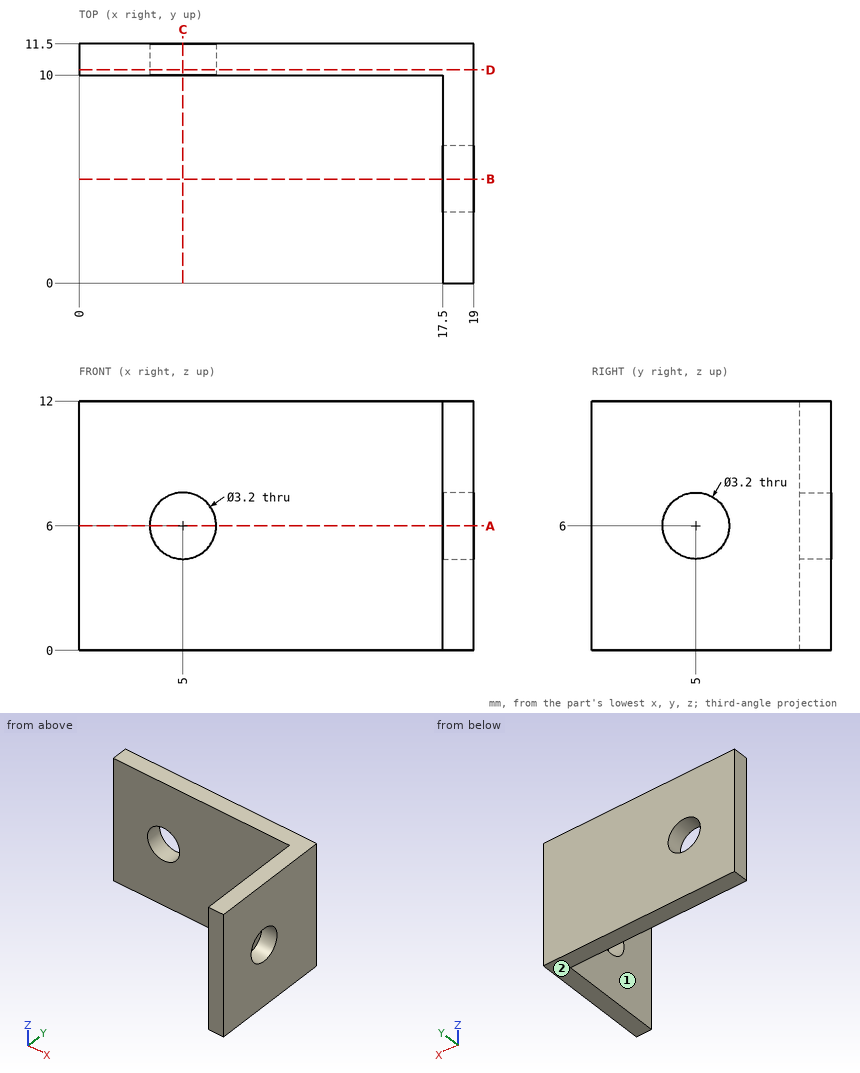
Part print with two shaded views. Sizes in mm from the minimum x, y, z corner. A direction names the side the tool comes from. Round coordinates to 2 decimals unless told otherwise and drop trailing zeros. Order: outer loops, then holes, each group sorted by start corner. A loop starts at its lowest first (then second) coordinate and runs counter-clockwise, first axis right, second up. Notation, with made-up numbers: M 83,11.25 L 128,11.25 A27 cw 128,35.25 Z; hole C -26,79 d4. An arc over 180 degrees is marked long. Answer in a Markdown table with one row per item. Add a question column.
Q1. 3-axis set-ups, long thin cutter, end or side, ignore diameter. For the marked faces 1 and 2: which of +Z, -Z, +X, -X, +Y, -Y reach the whole face in a straight line?
Q2. Wall check: L1, parallel to Z at x = 5, y = 10.6; L2, parallel to Y at x = 18.55, z = 6; L3, parallel to Y at x = 9, z = 5.5. Give the ranges that are in metal, low to high. Write a range as from..to.
Q3. Cut at A-A on z = 6. Give the cut face in (x, y).
Q4. Cut at C-C on x = 5. Give the cut face in (y, z), and give its area (3 significant figures).
Q5. Pin check, flat tips, straight feed: pin 1 (4 mm diameter, centred on x = 2, z = 4.5, fed in from -Y); pin 2 (3 mm diameter, centred on y = 3, z = 5, fed in from -X). Stop position of each tip, or through.
Q6. Cut at B-B on y = 5. Give the cut face in (x, z), and give its area (3 significant figures).
Q7. Cut at D-D on y = 10.25. Give the cut face in (x, z), and give its area (3 significant figures).
Established:
| question | item | result |
|---|---|---|
| 1 | face 1 | +Z, -Z, -X, -Y |
| 1 | face 2 | -Z, +X, -X, +Y, -Y |
| 2 | L1 | z = 0..4.4, 7.6..12 |
| 2 | L2 | y = 0..3.4, 6.6..11.5 |
| 2 | L3 | y = 10..11.5 |
| 3 | outline | M 0,10 L 3.4,10 L 3.4,11.5 L 0,11.5 Z; M 6.6,10 L 17.5,10 L 17.5,6.6 L 19,6.6 L 19,11.5 L 6.6,11.5 Z; M 17.5,0 L 19,0 L 19,3.4 L 17.5,3.4 Z |
| 4 | outline | M 10,0 L 11.5,0 L 11.5,4.4 L 10,4.4 Z; M 10,7.6 L 11.5,7.6 L 11.5,12 L 10,12 Z |
| 4 | area | 13.2 mm2 |
| 5 | pin 1 | stops at y = 10 |
| 5 | pin 2 | stops at x = 17.5 |
| 6 | outline | M 17.5,0 L 19,0 L 19,4.4 L 17.5,4.4 Z; M 17.5,7.6 L 19,7.6 L 19,12 L 17.5,12 Z |
| 6 | area | 13.2 mm2 |
| 7 | outline | M 0,0 L 19,0 L 19,12 L 0,12 Z; hole C 5,6 d3.2 |
| 7 | area | 220 mm2 |
